Print and shaded views of the part. All mm, measured from the part's lowest x, y and z. A direction names the side the tool comes from. Round coordinates to 2 decimals unless told otherwise and drop trailing zeros. Loops run counter-clockwise (first coordinate to the right, second up) from the corner with the lowest first, then second, coordinate; pieces in that order, holes last. Notation, with made-up numbers: (-12.5, 39) - (-1.5, 39) arc R22 cw to (-1.5, 66) - close; hole circle Ø8 at (43, 84). An arc over 180 degrees is marked (long way). Use one line per item in the form item = value. Start each with the question number.
Q1. Pin check, flat tips, straight feed: pin 1 (5 mm diameter, centred on x = 22, y = 14, fed in from +Z); pin 2 (5 mm diameter, centred on y = 14.5, z = 8.5, fed in from +X); pin 3 (3.5 mm diameter, centred on x = 13, z = 13.5, fed in from +Y); pin 4 (12 mm diameter, centred on x = 5, z = 11.5, fed in from +Y). Stop position of each tip, or through.
Q2. Saw through at A-A (z = 1.75). Give the cut face in (x, y).
Q3. Saw through at C-C (x = 9.5). Give the cut face in (y, z).
Q4. Saw through at B-B (y = 15.5). Give the cut face in (x, z).
Q5. Mould opens along Z. For the marked faces 1, 2 and 3 say: released by +Z, released by -Z, zero draft, split by the parting line, or undercut.
Q6. Saw through at D-D (x = 19.5). Give the cut face in (y, z).
Q7. 3-axis set-ups, long thin cutter, end or side, ignore diameter. For the marked faces 4 and 5: which of +Z, -Z, +X, -X, +Y, -Y reach the whole face in a straight line?
Q8. Drill centre lines: line 1 (Y direction, x = 8, z = 2.8); line 2 (Y direction, x = 7, z = 18.5). Where is each one in solid material? Low to high.
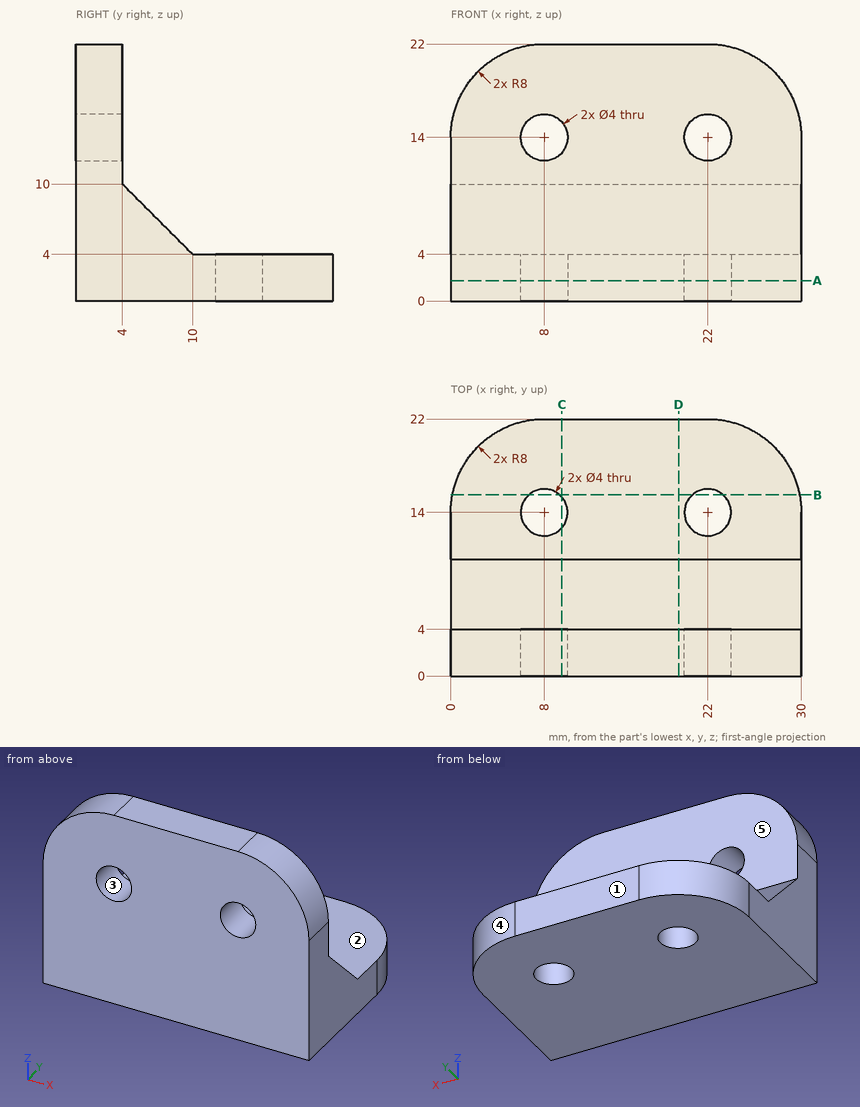
Report:
q1.pin_1 = 4
q1.pin_2 = through
q1.pin_3 = 4
q1.pin_4 = 8.5
q2.outline = (0, 0) - (30, 0) - (30, 14) arc R8 ccw to (22, 22) - (8, 22) arc R8 ccw to (0, 14) - close; hole circle Ø4 at (8, 14); hole circle Ø4 at (22, 14)
q3.outline = (0, 0) - (12.68, 0) - (12.68, 4) - (10, 4) - (4, 10) - (4, 12.68) - (0, 12.68) - close; (0, 15.32) - (4, 15.32) - (4, 22) - (0, 22) - close; (15.32, 0) - (22, 0) - (22, 4) - (15.32, 4) - close
q4.outline = (0.14, 0) - (6.68, 0) - (6.68, 4) - (0.14, 4) - close; (9.32, 0) - (20.68, 0) - (20.68, 4) - (9.32, 4) - close; (23.32, 0) - (29.86, 0) - (29.86, 4) - (23.32, 4) - close
q5.face_1 = zero draft
q5.face_2 = released by +Z
q5.face_3 = undercut
q6.outline = (0, 0) - (22, 0) - (22, 4) - (10, 4) - (4, 10) - (4, 22) - (0, 22) - close
q7.face_4 = +Z, -Z, +X, +Y
q7.face_5 = +Z, +X, -X, +Y
q8.line_1 = 0 to 12, 16 to 22
q8.line_2 = 0 to 4
